```python
from build123d import *
from build123d.topology import SkipClean

# Parameters (mm, degrees)
SKETCH1_R           = 2.35
BOSS_EXTRUDE1_DEPTH = 5
BOSS_EXTRUDE2_DEPTH = 13.4
BOSS_EXTRUDE3_START = 18.4
SKETCH1_2_R         = 2.35
BOSS_EXTRUDE3_DEPTH = 16.6
BOSS_EXTRUDE4_START = 30
SKETCH2_2_R         = 2.35
BOSS_EXTRUDE4_DEPTH = 13.4
BOSS_EXTRUDE5_START = 48.4
SKETCH1_3_R         = 2.35
BOSS_EXTRUDE5_DEPTH = 5
CHAMFER1_SIZE       = 3


with BuildPart() as part:
    # Sketch1 → Boss-Extrude1 (new body)
    with BuildSketch(Plane(origin=(0, 0, 0), x_dir=(1, 0, 0), z_dir=(0, 1, 0))):
        with Locations(Location((0, 0, 0), (0, 0, 270))):
            Circle(SKETCH1_R)
    extrude(amount=BOSS_EXTRUDE1_DEPTH)

    # Sketch2 → Boss-Extrude2 (add)
    with SkipClean():  # the faces are left unmerged after this step: merging them gives an invalid solid
        with BuildSketch(Plane(origin=(0, 5, 0), x_dir=(1, 0, 0), z_dir=(0, 1, 0))):
            with BuildLine():
                Line((-1.809005, -1.5), (-5.35, -1.5))
                Line((-5.35, -1.5), (-5.35, 1.5))
                Line((-5.35, 1.5), (-1.809005, 1.5))
                ThreePointArc((-1.809005, 1.5), (0, 2.35), (1.809005, 1.5))
                Line((1.809005, 1.5), (5.35, 1.5))
                Line((5.35, 1.5), (5.35, -1.5))
                Line((5.35, -1.5), (1.809005, -1.5))
                ThreePointArc((1.809005, -1.5), (0, -2.35), (-1.809005, -1.5))
            make_face()
        extrude(amount=BOSS_EXTRUDE2_DEPTH)

    # Sketch1<2> → Boss-Extrude3 (add)
    with SkipClean():  # the faces are left unmerged after this step: merging them gives an invalid solid
        with BuildSketch(Plane(origin=(0, 0, 0), x_dir=(1, 0, 0), z_dir=(0, 1, 0)).offset(BOSS_EXTRUDE3_START)):
            with Locations(Location((0, 0, 0), (0, 0, 270))):
                Circle(SKETCH1_2_R)
        extrude(amount=BOSS_EXTRUDE3_DEPTH)

    # Sketch2<2> → Boss-Extrude4 (add)
    with SkipClean():  # the faces are left unmerged after this step: merging them gives an invalid solid
        with BuildSketch(Plane(origin=(0, 5, 0), x_dir=(1, 0, 0), z_dir=(0, 1, 0)).offset(BOSS_EXTRUDE4_START)):
            with Locations(Location((0, 0, 0), (0, 0, 140.334987))):
                Circle(SKETCH2_2_R)
            with BuildLine():
                Line((-1.809005, -1.5), (-5.35, -1.5))
                Line((-5.35, -1.5), (-5.35, 1.5))
                Line((-5.35, 1.5), (-1.809005, 1.5))
                ThreePointArc((-1.809005, 1.5), (0, 2.35), (1.809005, 1.5))
                Line((1.809005, 1.5), (5.35, 1.5))
                Line((5.35, 1.5), (5.35, -1.5))
                Line((5.35, -1.5), (1.809005, -1.5))
                ThreePointArc((1.809005, -1.5), (0, -2.35), (-1.809005, -1.5))
            make_face()
        extrude(amount=BOSS_EXTRUDE4_DEPTH)

    # Sketch1<3> → Boss-Extrude5 (add)
    with SkipClean():  # the faces are left unmerged after this step: merging them gives an invalid solid
        with BuildSketch(Plane(origin=(0, 0, 0), x_dir=(1, 0, 0), z_dir=(0, 1, 0)).offset(BOSS_EXTRUDE5_START)):
            with Locations(Location((0, 0, 0), (0, 0, 270))):
                Circle(SKETCH1_3_R)
        extrude(amount=BOSS_EXTRUDE5_DEPTH)

    # Chamfer1
    # the kernel refuses this chamfer: 3 mm, written as the material it adds along each edge
    with BuildSketch(Plane(origin=(0, 18.4, 0), x_dir=(0.9999950652018581, 0, -0.0031415874858791225), z_dir=(0.0031415874858791225, 0, 0.9999950652018581))) as chamfer1_piece_1_section:
        Polygon((2.35, CHAMFER1_SIZE), (2.35 + CHAMFER1_SIZE, 0), (2.35, 0), align=None)
    chamfer1_piece_1 = revolve(axis=Axis((0, 18.4, 0), (0, 1, 0)), revolution_arc=359.64, mode=Mode.PRIVATE)
    chamfer1_piece_1 = split(chamfer1_piece_1, bisect_by=Plane(origin=(3.194483, 19.397878, 1.5), z_dir=(0, 0, -1)), keep=Keep.TOP, mode=Mode.PRIVATE)
    chamfer1_piece_1 = split(chamfer1_piece_1, bisect_by=Plane(origin=(3.194483, 19.397878, -1.5), z_dir=(0, 0, 1)), keep=Keep.TOP, mode=Mode.PRIVATE)
    chamfer1_piece_1 = split(chamfer1_piece_1, bisect_by=Plane(origin=(-5.35, 19.397878, -0.77195), z_dir=(1, 0, 0)), keep=Keep.TOP, mode=Mode.PRIVATE)
    add(chamfer1_piece_1)
    with BuildSketch(Plane(origin=(0, 18.4, 0), x_dir=(-0.9999950652018581, 0, 0.0031415874858796884), z_dir=(-0.0031415874858796884, 0, -0.9999950652018581))) as chamfer1_piece_2_section:
        Polygon((2.35, CHAMFER1_SIZE), (2.35 + CHAMFER1_SIZE, 0), (2.35, 0), align=None)
    chamfer1_piece_2 = revolve(axis=Axis((0, 18.4, 0), (0, 1, 0)), revolution_arc=359.64, mode=Mode.PRIVATE)
    chamfer1_piece_2 = split(chamfer1_piece_2, bisect_by=Plane(origin=(-3.194483, 19.397878, 1.5), z_dir=(0, 0, -1)), keep=Keep.TOP, mode=Mode.PRIVATE)
    chamfer1_piece_2 = split(chamfer1_piece_2, bisect_by=Plane(origin=(-3.194483, 19.397878, -1.5), z_dir=(0, 0, 1)), keep=Keep.TOP, mode=Mode.PRIVATE)
    chamfer1_piece_2 = split(chamfer1_piece_2, bisect_by=Plane(origin=(5.35, 19.397878, 0.77195), z_dir=(-1, 0, 0)), keep=Keep.TOP, mode=Mode.PRIVATE)
    add(chamfer1_piece_2)
    with BuildSketch(Plane(origin=(0, 35, 0), x_dir=(-0.9999950652018581, 0, 0.0031415874858796884), z_dir=(-0.0031415874858796884, 0, -0.9999950652018581))) as chamfer1_piece_3_section:
        Polygon((2.35, -CHAMFER1_SIZE), (2.35 + CHAMFER1_SIZE, 0), (2.35, 0), align=None)
    chamfer1_piece_3 = revolve(axis=Axis((0, 35, 0), (0, 1, 0)), revolution_arc=359.64, mode=Mode.PRIVATE)
    chamfer1_piece_3 = split(chamfer1_piece_3, bisect_by=Plane(origin=(-3.194483, 34.002122, 1.5), z_dir=(0, 0, -1)), keep=Keep.TOP, mode=Mode.PRIVATE)
    chamfer1_piece_3 = split(chamfer1_piece_3, bisect_by=Plane(origin=(-3.194483, 34.002122, -1.5), z_dir=(0, 0, 1)), keep=Keep.TOP, mode=Mode.PRIVATE)
    chamfer1_piece_3 = split(chamfer1_piece_3, bisect_by=Plane(origin=(5.35, 34.002122, 0.77195), z_dir=(-1, 0, 0)), keep=Keep.TOP, mode=Mode.PRIVATE)
    add(chamfer1_piece_3)
    with BuildSketch(Plane(origin=(0, 35, 0), x_dir=(0.9999950652018625, 0, -0.0031415874844589325), z_dir=(0.0031415874844589325, 0, 0.9999950652018625))) as chamfer1_piece_4_section:
        Polygon((2.35, -CHAMFER1_SIZE), (2.35 + CHAMFER1_SIZE, 0), (2.35, 0), align=None)
    chamfer1_piece_4 = revolve(axis=Axis((0, 35, 0), (0, 1, 0)), revolution_arc=359.64, mode=Mode.PRIVATE)
    chamfer1_piece_4 = split(chamfer1_piece_4, bisect_by=Plane(origin=(3.194483, 34.002122, 1.5), z_dir=(0, 0, -1)), keep=Keep.TOP, mode=Mode.PRIVATE)
    chamfer1_piece_4 = split(chamfer1_piece_4, bisect_by=Plane(origin=(-5.35, 34.002122, -0.77195), z_dir=(1, 0, 0)), keep=Keep.TOP, mode=Mode.PRIVATE)
    chamfer1_piece_4 = split(chamfer1_piece_4, bisect_by=Plane(origin=(3.194483, 34.002122, -1.5), z_dir=(0, 0, 1)), keep=Keep.TOP, mode=Mode.PRIVATE)
    add(chamfer1_piece_4)


solid = part.part
```
Geometry check sheet. Reference: the model listing, model coordinates, mm. A direction names the side the tool comes from. Give positions to 0.01 mm unless a question says otherwise; leave off trailing zeros. Loops run counter-clockwise (first coordinate to the right, second up) from the corner with the lowest first, then second, coordinate; pieces in that order, holes last. Notation, with made-up numbers: M 87.25,64 L 111.25,64 A21 cw 111.25,90 Z; hole C 79.25,-16 d3. An arc over 180 degrees is marked long. Answer as CSV lines item,"result".
Item 1: Release check for a two-part mould opening along Y. For faces 4 (the conical face through (3.54, 33.19, 0.03)), 5 (the flat face through (4, 48.4, 0)), 6 (the flat face through (4, 13, 1.5)), 7 (the conical face through (3.54, 20.21, 0.03)) record: pulls with the +Y half, pulls with the -Y half, needs draft (parallel to the pull), parting line crosses it, or undercut.
Values:
face 4,"undercut"
face 5,"pulls with the +Y half"
face 6,"needs draft"
face 7,"undercut"
Item 2: Access from +Z, -Z, +X, -X, +Y, -Y to the whole of each face (thin tool, end or side, straight path). Record for faces 1 (the flat face through (4, 40, 1.5)), 2 (the flat face through (-4, 13, -1.5)), 3 (the conical face through (-3.54, 33.19, -0.03)).
Values:
face 1,"+Z, +X, +Y, -Y"
face 2,"-Z, -X, +Y, -Y"
face 3,"-X"
Item 3: Depth check by flat-ended pin: P1, Ø1.8, axis at x = 3.5, y = 12, coming from the +Z side; P2, Ø1.1, axis at x = -3.5, y = 12, coming from the -Z side; P3, Ø0.9, axis at x = -4, z = 0, coming from the -Y side. Enter the tip coordinate at first touch or a pass-through.
Values:
P1,"stops at z = 1.5"
P2,"stops at z = -1.5"
P3,"stops at y = 5"
Item 4: Material ranges on line 1 (X direction, y = 5.5, z = 1.8); line 2 (Z direction, x = 2.75, y = 38); line 3 (Y direction, x = 4.25, z = -0.7), recorded low to high.
Values:
line 1,"x = -1.51 to 1.51"
line 2,"z = -1.5 to 1.5"
line 3,"y = 5 to 19.44, 33.96 to 48.4"
Item 5: Cross-section at A-A on x = 1. Record the cut outline in (y, z).
Values:
outline,"M 0,-2.13 L 53.4,-2.13 L 53.4,2.13 L 0,2.13 Z"
